Autodesk Inventor part; units mm, degrees
ref_plane "YZ Plane" through (0, 0, 0) normal (1, 0, 0) x (0, 1, 0)
ref_plane "XZ Plane" through (0, 0, 0) normal (0, 1, 0) x (-1, 0, 0)
ref_plane "XY Plane" through (0, 0, 0) normal (0, 0, 1) x (1, 0, 0)
sketch "Skizze1" plane through (0, 0, 0) normal (0, 1, 0) x (-1, 0, 0)
  line L0 (0, 0) -> (0, 6.5)
  line L1 (0, 6.5) -> (-10.5, 6.5)
  line L2 (-10.5, 6.5) -> (-10.5, 5)
  line L3 (-10.5, 5) -> (-28.5, 5)
  line L4 (-28.5, 5) -> (-28.5, 3)
  line L5 (-28.5, 3) -> (-46.5, 3)
  line L6 (-46.5, 3) -> (-46.5, 0)
  line L7 (-46.5, 0) -> (0, 0)
  dimension "d0" = 46.5
  dimension "d1" = 13
  dimension "d2" = 10
  dimension "d3" = 6
  dimension "d4" = 10.5
  dimension "d5" = 18
revolve "Umdrehung1" add sketch "Skizze1" angle 360 about axis through (46.5, 0, 0) along (-1, 0, 0)
thread "Gewinde1"
sketch "Skizze2" plane through (0, 0, 0) normal (-1, 0, 0) x (0, 0, 1)
  circle A0 centre (0, 0) radius 6.5
  point P0 (0, 0)
hole "Bohrung1" at (0, 0, 0) direction (1, 0, 0) diameter 4 depth 26
chamfer "Fasen1" distance 0.35 angle 45 2 edges at (28.5, 0, -5) (10.5, 0, -6.5)
properties part number "102" material "Silber"
Build history of the part. All positions in model axes, mm. A direction names the side the tool comes from. Coordinates: 2 decimals unless noted, no trailing zeros. Order: outer loops, then holes, each group sorted by start corner. A loop starts at its lowest first (then second) coordinate and runs counter-clockwise, first axis right, second up. Notation, with made-up numbers: (28.25, -7.5) - (41.25, -7.5) arc R23 ccw to (41.25, 9.5) - close; hole circle Ø3 at (80.25, -6). An arc over 180 degrees is marked (long way). Write item = value, one per line. Start each with the question number.
1) Two-plate mould, pull along Z, no slides. Class faces 1 (the face through (13, 2, 0)), 2 (the face through (38, 0, -3)), 3 (the face through (10.5, 5, -2)), 4 (the face through (26, 0, 0)): pulls with the +Z half, pulls with the -Z half, needs draft (parallel to the pull), parting line crosses it, or undercut.
2) Saw through at A-A on y = 0. Write the cut outline in (x, z).
3) Flat gauge pins, fed straight in: pin 1 Ø2.5 at (y, z) = (0, 0) entering from -X; pin 2 Ø1.5 at (x, z) = (36.5, -5) entering from +Y; pin 3 Ø2 at (x, z) = (40.5, -0.5) entering from +Y; pin 4 Ø3 at (y, z) = (2, 5) entering from +X. Where does each tip first touch, or does it go through?
4) Saw through at D-D on x = 27. Write the cut outline in (y, z), then the cut area to 3 significant figures.
5) 3-axis set-ups, long thin cutter, end or side, ignore diameter. For faces 5 (the face through (46.5, 0, 0)), 6 (the face through (19.45, 4.88, -1.08)): which of +Z, -Z, +X, -X, +Y, -Y reach the whole face in a straight line?
6) Saw through at C-C on x = 6. Write the cut outline in (y, z), then the cut area to 3 significant figures.
7) Wall check: line 1 along Y through (x, z) = (8.5, 0); line 2 along X through (y, z) = (-5.5, -2.5); line 3 along X through (y, z) = (-3.25, 1.5). Give the ranges that are in metal, low to high. Write a range as from..to.
From the geometry:
q1.face_1 = undercut
q1.face_2 = parting line crosses it
q1.face_3 = needs draft
q1.face_4 = undercut
q2.outline = (0, -6.5) - (10.15, -6.5) - (10.5, -6.15) - (10.5, -5) - (28.15, -5) - (28.5, -4.65) - (28.5, -3) - (46.5, -3) - (46.5, 3) - (28.5, 3) - (28.5, 4.65) - (28.15, 5) - (10.5, 5) - (10.5, 6.15) - (10.15, 6.5) - (0, 6.5) - (0, 2) - (26, 2) - (26, -2) - (0, -2) - close
q3.pin_1 = 26
q3.pin_2 = through
q3.pin_3 = 3
q3.pin_4 = 28.5
q4.outline = circle Ø10 at (0, 0)
q4.area = 78.5 mm^2
q5.face_5 = +Z, -Z, +X, +Y, -Y
q5.face_6 = +X
q6.outline = circle Ø13 at (0, 0); hole circle Ø4 at (0, 0)
q6.area = 120 mm^2
q7.line_1 = -6.5..-2, 2..6.5
q7.line_2 = 0..10.5
q7.line_3 = 0..28.5
